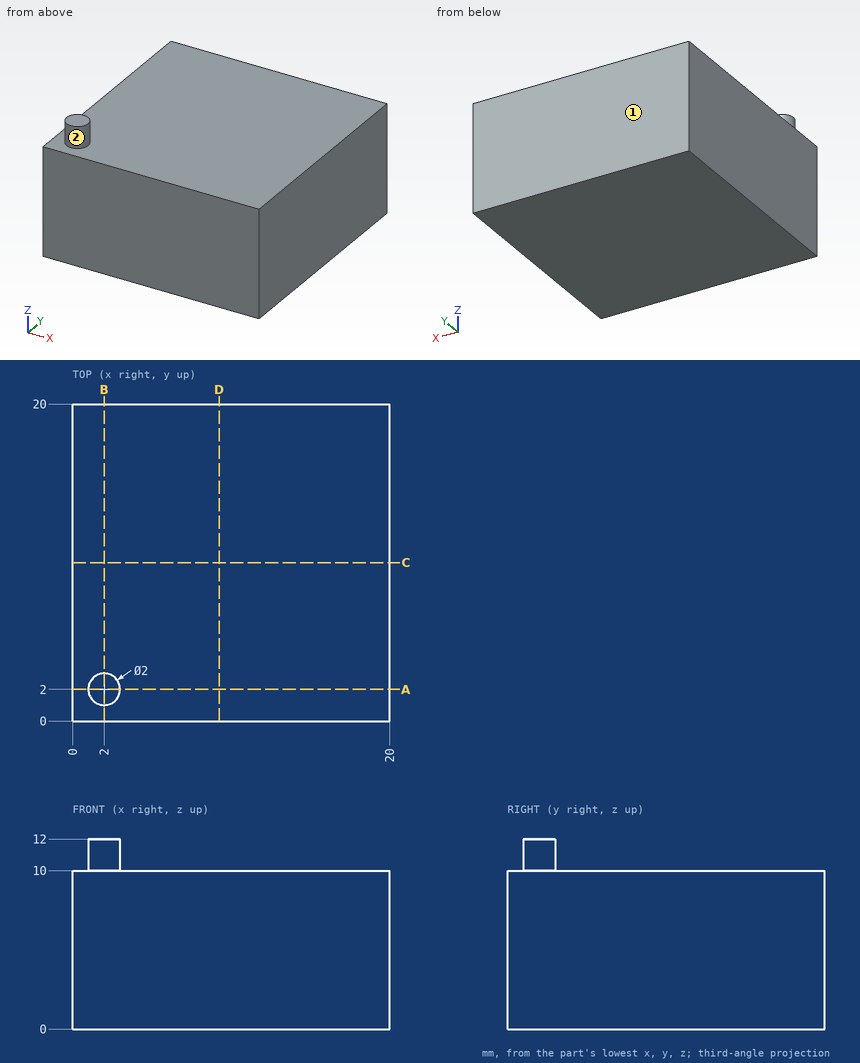
Job drawing, mm, ordinate dimensions from the low corner. One solid piece. A direction names the side the tool comes from. Coordinates: 2 decimals unless noted, no trailing zeros. Loops run counter-clockwise (first coordinate to the right, second up) from the corner with the lowest first, then second, coordinate; pieces in that order, holes last. Notation, with made-up numbers: (-8, 29.25) - (45, 29.25) arc R10 ccw to (45, 39.25) - close; hole circle Ø3 at (51.5, -24.5). An arc over 180 degrees is marked (long way). Write item = value, one per line. Start each with the question number.
Q1. Drill centre line: L1, parallel to Z at x = 13.25, y = 13. Where is it in solid material? Low to high.
Q2. Cut at A-A, the plane y = 2. List the corners of the cut face in (x, z).
Q3. Flat gauge pin, fed straight in: pin 1 Ø5 at (x, y) = (6, 6.5) entering from +Z. Where does the tip first touch, or does it go through?
Q4. Which spindle directions (+Z, -Z, +X, -X, +Y, -Y) get a long thin tool onto all of the face, cutting with end or side? Do the marked faces 1 and 2. Say none if no direction does.
Q5. Cut at C-C, the plane y = 10. List the corners of the cut face in (x, z), then the cut area to 3 significant figures.
Computed:
q1.L1 = 0 to 10
q2.outline = (0, 0) - (20, 0) - (20, 10) - (3, 10) - (3, 12) - (1, 12) - (1, 10) - (0, 10) - close
q3.pin_1 = 10
q4.face_1 = +Z, -Z, +X, -X, +Y
q4.face_2 = +Z
q5.outline = (0, 0) - (20, 0) - (20, 10) - (0, 10) - close
q5.area = 200 mm²
